Geometry check sheet. Reference: drawing and pictorial views, mm from the part's lowest x, y, z. A direction names the side the tool comes from. Coordinates: 2 decimals unless noted, no trailing zeros. Loops run counter-clockwise (first coordinate to the right, second up) from the corner with the lowest first, then second, coordinate; pieces in that order, holes last. Notation, with made-up numbers: (-31.5, 88) -> (-15.5, 88) arc R14 ccw to (-15.5, 104) -> close; hole circle Ø7 at (27.25, -37). An arc over 180 degrees is marked (long way). Answer as a JSON object with one key per item and string values. Group by question number.
Q1. Scan lines: L1, parallel to Z at x = 33.5, y = 21; L2, parallel to Y at x = 18, z = 64; L3, parallel to Y at x = 18.5, z = 36.5 (1 decimal). Record each from-to range of solid material in increasing order.
Q2. Set-up check for the marked faces 1 and 2: record each of +Z, -Z, +X, -X, +Y, -Y from which the full face is reachable in a straight line by a thin tool's end or side.
Q3. Cross-section at C-C on x = 4.5. Record the boundary of the cut face in (y, z), and give its area (3 significant figures).
Q4. Cross-section at D-D on z = 8. Record the boundary of the cut face in (x, y), and give its area (3 significant figures).
Q5. Cross-section at A-A on y = 12.5. Record the boundary of the cut face in (x, z) (1 decimal).
Q6. Gauge pin test, flat ends, axial feed: pin 1 Ø5.5 at (x, y) = (17.78, 5.4) entering from +Z; pin 2 Ø1.5 at (x, z) = (13, 44) entering from +Y; pin 3 Ø5 at (x, z) = (6, 52) entering from -Y (1 decimal). Record the tip position at first contact, or that the pin passes through.
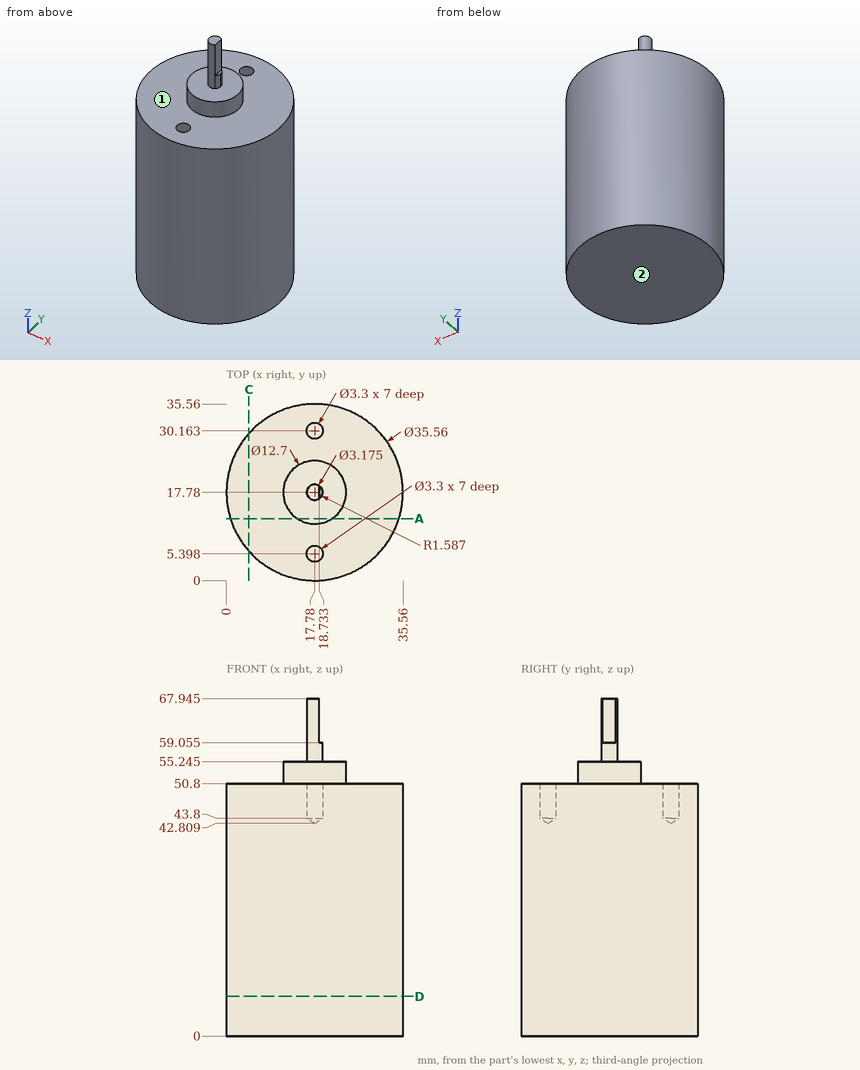
Computed values:
{
 "1": {"L1": "z = 0 to 50.8", "L2": "y = 16.21 to 19.35", "L3": "y = 0 to 35.5"},
 "2": {"face 1": "+Z", "face 2": "-Z, +X, -X, +Y, -Y"},
 "3": {"outline": "(5.96, 0) -> (29.6, 0) -> (29.6, 50.8) -> (5.96, 50.8) -> close", "area": "1,200 mm²"},
 "4": {"outline": "circle Ø35.56 at (17.78, 17.78)", "area": "993 mm²"},
 "5": {"outline": "(0.8, 0) -> (34.8, 0) -> (34.8, 50.8) -> (21.3, 50.8) -> (21.3, 55.2) -> (14.3, 55.2) -> (14.3, 50.8) -> (0.8, 50.8) -> close"},
 "6": {"pin 1": "stops at z = 50.8", "pin 2": "stops at y = 35.1", "pin 3": "stops at y = 2.8"}
}
